from build123d import *

# Parameters (mm, degrees)
F0_W      = 70
F0_H      = 130
F1_DEPTH  = 0.8
F2_SIZE   = 5
F3_W      = 50
F3_H      = 0.8
F4_DEPTH  = 3
F5_W      = 50
F5_H      = 0.8
F6_ANGLE  = 90
F7_DEPTH  = 17.5
F8_W      = 50
F8_H      = 0.8
F9_ANGLE  = 90
F10_DEPTH = 25
F11_R     = 2


with BuildPart() as f1:
    # F0 (on Top) → F1 (new body)
    with BuildSketch(Plane.XY):
        with Locations((-5.7087102905, -38.4061143195)):
            Rectangle(F0_W, F0_H)
    extrude(amount=F1_DEPTH)

    # F2
    f2_edges = [f1.edges().sort_by_distance(p)[0] for p in [
        (-40.70871, -103.406114, 0.4),
        (29.29129, -103.406114, 0.4),
        (29.29129, 26.593886, 0.4),
        (-40.70871, 26.593886, 0.4),
    ]]
    chamfer(f2_edges, length=F2_SIZE)

    # F3 (on face) → F4 (join)
    with BuildSketch(Plane(origin=(0, 26.5938856805, 0), x_dir=(-1, 0, 0), z_dir=(0, 1, 0))):
        with Locations((5.7087102905, 0.4)):
            Rectangle(F3_W, F3_H)
    extrude(amount=F4_DEPTH)

    # F5 (on face) → F6 (revolve)
    with BuildSketch(Plane(origin=(0, 29.5938856805, 0), x_dir=(-1, 0, 0), z_dir=(0, 1, 0))):
        with Locations((5.7087102905, 0.4)):
            Rectangle(F5_W, F5_H)
    revolve(axis=Axis((-7.0197554305, 29.5938856805, -1.5), (-1, 0, 0)), revolution_arc=F6_ANGLE)

    # F7 (add): a face of the model
    f7_faces = [f1.faces().sort_by_distance(p)[0] for p in [
        (-5.7087102905, 31.4938856805, -1.5),
    ]]
    extrude(f7_faces, amount=F7_DEPTH)

    # F8 (on face) → F9 (revolve)
    with BuildSketch(Plane(origin=(0, 0, -19), x_dir=(1, 0, 0), z_dir=(0, 0, -1))):
        with Locations((-5.7087102905, -31.4938856805)):
            Rectangle(F8_W, F8_H)
    revolve(axis=Axis((-5.6677348912, 30.3438856805, -19), (-1, 0, 0)), revolution_arc=F9_ANGLE)

    # F10 (add): a face of the model
    f10_faces = [f1.faces().sort_by_distance(p)[0] for p in [
        (-5.7087102905, 30.3438856805, -20.15),
    ]]
    extrude(f10_faces, amount=F10_DEPTH)

    # F11
    f11_edges = [f1.edges().sort_by_distance(p)[0] for p in [
        (-30.70871, 26.593886, 0.4),
        (19.29129, 26.593886, 0.4),
    ]]
    fillet(f11_edges, radius=F11_R)


solid = f1.part
Source: CAD feature listing. Evaluate the final solid. Frame: model axes, mm. A direction names the side the tool comes from. Coordinates: 2 decimals unless noted, no trailing zeros. Loops run counter-clockwise (first coordinate to the right, second up) from the corner with the lowest first, then second, coordinate; pieces in that order, holes last. Notation, with made-up numbers: M 56,44.5 L 60,44.5 A4 ccw 60,50.5 Z; hole C 86.5,86.25 d8. An arc over 180 degrees is marked long. Answer in a Markdown table with one row per item.
Q1. Section A-A on y = 19. Return the cut outline in (x, z).
Answers below:
| item | result |
|---|---|
| outline | M -40.71,0 L 29.29,0 L 29.29,0.8 L -40.71,0.8 Z; M -30.71,-20.55 L 19.29,-20.55 L 19.29,-19.75 L -30.71,-19.75 Z |
Q2. Section C-C on z = -14.5. Return the cut outline in (x, y), plus the area to 3 significant figures.
Answers below:
| item | result |
|---|---|
| outline | M -30.71,31.09 L 19.29,31.09 L 19.29,31.89 L -30.71,31.89 Z |
| area | 40.0 mm^2 |
Q3. First-contact query: pin 1 (8 mm diameter, centred on y = 17, z = -12.5, fed in from -X); pin 2 (0.9 mm diameter, centred on x = 23, z = 0.5, fed in from +Y); pin 3 (9 mm diameter, centred on x = 5.5, z = -14.5, fed in from -Y); pin 4 (6 mm diameter, centred on x = 12, y = -30, fed in from -Z). Flat tips, straight axial feed; report the tip coordinate or a pass-through.
Answers below:
| item | result |
|---|---|
| pin 1 | passes through |
| pin 2 | stops at y = 26.59 |
| pin 3 | stops at y = 31.09 |
| pin 4 | stops at z = 0 |
Q4. Section B-B on x = -7. Return the cut outline in (y, z).
Answers below:
| item | result |
|---|---|
| outline | M -103.41,0 L 29.59,0 A1.5 cw 31.09,-1.5 L 31.09,-19 A0.75 cw 30.34,-19.75 L 5.34,-19.75 L 5.34,-20.55 L 30.34,-20.55 A1.55 ccw 31.89,-19 L 31.89,-1.5 A2.3 ccw 29.59,0.8 L -103.41,0.8 Z |
Q5. Section D-D on y = -24. Return the cut outline in (x, z), plus the area to 3 significant figures.
Answers below:
| item | result |
|---|---|
| outline | M -40.71,0 L 29.29,0 L 29.29,0.8 L -40.71,0.8 Z |
| area | 56.0 mm^2 |
Q6. Ray query, probe 1 along Z at (x, y) = (-30, -53.5); probe 2 along Y at (x, z) = (2, -6). Return the intervals inside material, ascending. Write a range as from..to.
Answers below:
| item | result |
|---|---|
| probe 1 | z = 0..0.8 |
| probe 2 | y = 31.09..31.89 |
Q7. Set-up query: faces 1 (the flat face through (26.756, 24.129, 0.394)), 2 (the flat face through (-5, 31.094, -10)). Return all of +Z, -Z, +X, -X, +Y, -Y with unobstructed straight access to the full face (end or side cutting, diameter ignored); none if empty.
Answers below:
| item | result |
|---|---|
| face 1 | +Z, -Z, +X, +Y |
| face 2 | +X, -X, -Y |
Q8. Draft query along Z for faces 3 (the flat face through (26.8, -100.9, 0.4)), 4 (the flat face through (-6, 18, -19.75)), 5 (the flat face through (-6, 18, -20.55)). Return one class per face: pulls with the +Z half, pulls with the -Z half, needs draft (parallel to the pull), parting line crosses it, or undercut.
Answers below:
| item | result |
|---|---|
| face 3 | needs draft |
| face 4 | undercut |
| face 5 | pulls with the -Z half |
